Geometry: see drawing. Coordinates: mm, zero at the bounding-box minimum. Give positions to 0.01 mm unless a question says otherwise; leave off trailing zeros. Write each loop counter-clockwise with the first axis right and the second up, starting at its lowest first coordinate (ties: lowest second). Pieces come first, ordered by that corner, then holes. Notation, with made-up numbers: M -24,-21.5 L 35,-21.5 A10 cw 35,-12.5 Z; hole C 53,39 d8. An arc over 180 degrees is marked long. Use one line per item in the form item = value. Start each with the question number.
Item 1: Section query C-C on z = 5. Return loops of the section in (x, y) (3 decimals), then the cut area to 3 significant figures.
Item 2: Section query B-B on x = 292.1. Return loops of the section in (y, z) (3 decimals), then the cut area to 3 significant figures.
Item 3: Section query D-D on y = 17. Return loops of the section in (x, z).
Item 4: Contact query for flat-ended pins moving along their axis: P1, Ø4, axis at y = 11, z = 6.5, coming from the -X side; P2, Ø4, axis at y = 12, z = 8, coming from the +X side; P3, Ø6.5, axis at x = 466, z = 9, coming from the -Y side. Output: stop coordinate, or through.
Item 5: Material intervals for line 1 along Y through (x, z) = (292.1, 3.5) (3 decimals); line 2 along X through (y, z) = (52, 1.25); line 3 along X through (y, z) = (48, 9), sorted ascending. Write a range as from..to.
Item 6: Section query A-A on y = 51.5. Return loops of the section in (x, z) (3 decimals), then the cut area to 3 significant figures.
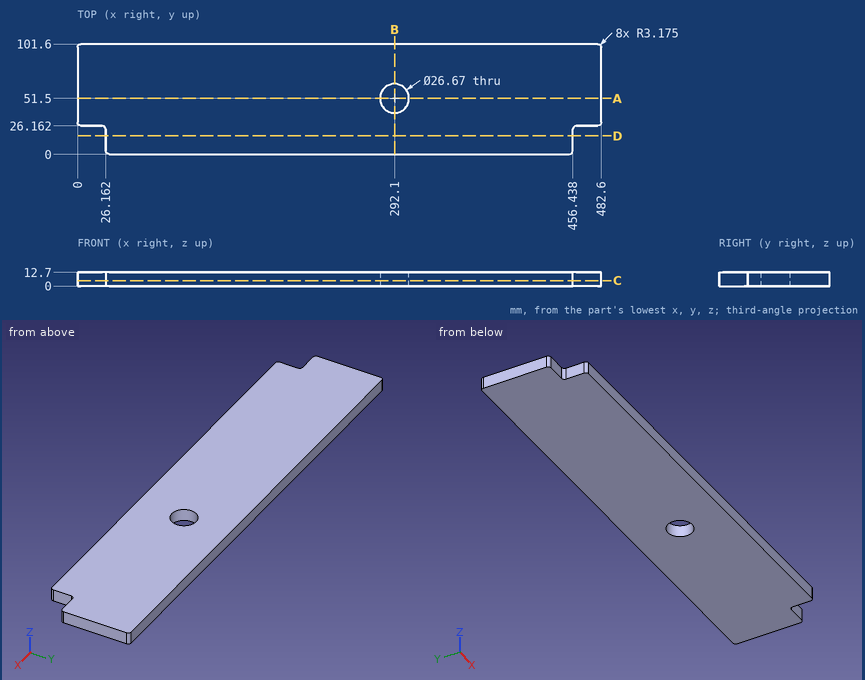
Answer sheet:
q1.outline = M 0,29.337 A3.175 ccw 3.175,26.162 L 22.987,26.162 A3.175 cw 26.162,22.987 L 26.162,3.175 A3.175 ccw 29.337,0 L 453.263,0 A3.175 ccw 456.438,3.175 L 456.438,22.987 A3.175 cw 459.613,26.162 L 479.425,26.162 A3.175 ccw 482.6,29.337 L 482.6,98.425 A3.175 ccw 479.425,101.6 L 3.175,101.6 A3.175 ccw 0,98.425 Z; hole C 292.1,51.5 d26.67
q1.area = 47,100 mm2
q2.outline = M 0,0 L 38.165,0 L 38.165,12.7 L 0,12.7 Z; M 64.835,0 L 101.6,0 L 101.6,12.7 L 64.835,12.7 Z
q2.area = 952 mm2
q3.outline = M 26.16,0 L 456.44,0 L 456.44,12.7 L 26.16,12.7 Z
q4.P1 = 26.16
q4.P2 = 456.44
q4.P3 = 26.16
q5.line_1 = 0..38.165, 64.835..101.6
q5.line_2 = 0..278.77, 305.43..482.6
q5.line_3 = 0..279.23, 304.97..482.6
q6.outline = M 0,0 L 278.765,0 L 278.765,12.7 L 0,12.7 Z; M 305.435,0 L 482.6,0 L 482.6,12.7 L 305.435,12.7 Z
q6.area = 5,790 mm2
